```python
from build123d import *

# Parameters (mm, degrees)
F1_DEPTH = 101.6


with BuildPart() as f1:
    # F0 (on Top) → F1 (new body)
    with BuildSketch(Plane.XY):
        with BuildLine():
            Line((-89.186773, -0.016751), (88.613227, -0.016751))
            Line((88.613227, -0.016751), (88.613227, 53.069249))
            Line((88.613227, 53.069249), (86.358745, 53.069249))
            ThreePointArc((86.358745, 53.069249), (84.106649, 52.18205), (83.064762, 49.997207))
            Line((83.064762, 49.997207), (80.458159, 12.659636))
            ThreePointArc((80.458159, 12.659636), (77.973661, 7.449628), (72.603276, 5.334))
            Line((72.603276, 5.334), (-69.297198, 5.334))
            ThreePointArc((-69.297198, 5.334), (-74.391767, 7.204231), (-77.066214, 11.926489))
            Line((-77.066214, 11.926489), (-83.396749, 50.304656))
            ThreePointArc((-83.396749, 50.304656), (-84.518291, 52.284958), (-86.654724, 53.069249))
            Line((-86.654724, 53.069249), (-89.186773, 53.069249))
            Line((-89.186773, 53.069249), (-89.186773, -0.016751))
        make_face()
    extrude(amount=F1_DEPTH)


solid = f1.part
```
Check sheet for the modelled part. Datum: model origin and axes. Units: mm. A direction names the side the tool comes from. Give positions to 0.01 mm unless a question says otherwise; leave off trailing zeros. Write each loop counter-clockwise with the first axis right and the second up, starting at its lowest first coordinate (ties: lowest second). Pieces come first, ordered by that corner, then holes. Notation, with made-up numbers: (36.25, -10) - (49.25, -10) arc R20 ccw to (49.25, 12) - close; hole circle Ø9 at (56.25, -19.5). An arc over 180 degrees is marked (long way). Answer as a JSON object with one key per item and string values. Group by question number.
1) Sectioned sample at C-C (y = 25). Record the cut outline in (x, z).
2) Sectioned sample at A-A (y = 16). Record the cut outline in (x, z), then the cut area to 3 significant figures.
3) Sectioned sample at D-D (x = -25). Record the cut outline in (y, z), then the cut area to 3 significant figures.
4) Sectioned sample at B-B (z = 70.5). Record the cut outline in (x, y).
5) Release check for a two-part mould opening along X. For faces 3 (the face through (-89.187, 27, 50)), 4 (the face through (-7, 5, 0)), 5 (the face through (84.132, 52.206, 50.089)), 6 (the face through (-80.187, 30.847, 50.089)) record: pulls with the +X half, pulls with the -X half, needs draft (parallel to the pull), parting line crosses it, or undercut.
6) Access from +Z, -Z, +X, -X, +Y, -Y to the whole of each face (thin tool, end or side, straight path). Record for faces 1 (the face through (81.78, 31.59, 50.09)), 2 (the face through (88.613, 26, 50)).
7) Thickness scan on probe 1 along Y at (x, z) = (52, 92); probe 2 along X at (y, z) = (10.5, 41); probe 3 along X at (y, z) = (33.5, 39.5). Record the ranges inside material, lowest first. Write a range as from..to.
Geometry results:
{
 "1": {"outline": "(-89.19, 0) - (-79.22, 0) - (-79.22, 101.6) - (-89.19, 101.6) - close; (81.32, 0) - (88.61, 0) - (88.61, 101.6) - (81.32, 101.6) - close"},
 "2": {"outline": "(-89.19, 0) - (-77.74, 0) - (-77.74, 101.6) - (-89.19, 101.6) - close; (80.69, 0) - (88.61, 0) - (88.61, 101.6) - (80.69, 101.6) - close", "area": "1,970 mm^2"},
 "3": {"outline": "(-0.02, 0) - (5.33, 0) - (5.33, 101.6) - (-0.02, 101.6) - close", "area": "544 mm^2"},
 "4": {"outline": "(-89.19, -0.02) - (88.61, -0.02) - (88.61, 53.07) - (86.36, 53.07) arc R3.3 ccw to (83.06, 50) - (80.46, 12.66) arc R7.87 cw to (72.6, 5.33) - (-69.3, 5.33) arc R7.87 cw to (-77.07, 11.93) - (-83.4, 50.3) arc R3.3 ccw to (-86.65, 53.07) - (-89.19, 53.07) - close"},
 "5": {"face 3": "pulls with the -X half", "face 4": "needs draft", "face 5": "undercut", "face 6": "undercut"},
 "6": {"face 1": "+Z, -Z, +Y", "face 2": "+Z, -Z, +X, +Y, -Y"},
 "7": {"probe 1": "y = -0.02..5.33", "probe 2": "x = -89.19..-76.69, 80..88.61", "probe 3": "x = -89.19..-80.62, 81.91..88.61"}
}
